Check sheet for the modelled part. Datum: model origin and axes. Units: mm. Face numbers are marked on the shaded views. A direction names the side the tool comes from. Give positions to 0.01 mm unless a question says otherwise; leave off trailing zeros. Loops run counter-clockwise (first coordinate to the right, second up) from the corner with the lowest first, then second, coordinate; pieces in that order, holes last. Notation, with made-up numbers: (54, 66) - (97, 66) arc R23 cw to (97, 74) - close; hole circle Ø7 at (-31, -24). An arc over 180 degrees is marked (long way). Answer in a Markdown table with one row per item. Add a question column.
(1) Set-up check for the marked faces 1 and 2: record each of +Z, -Z, +X, -X, +Y, -Y from which the full face is reachable in a straight line by a thin tool's end or side.
(2) Sectioned sample at A-A on y = 75. Enter the section's corners in (x, z).
(3) Go/stop test with flat-tipped pins: P1, Ø3, axis at x = 37.5, z = -37.5, coming from the +Y side; P2, Ø10, axis at x = 13.5, y = 96.5, coming from the +Z side; P3, Ø2.5, axis at x = 2.24, z = -37.13, coming from the +Y side. Record where each tip stops, or that it passes through.
(4) Sectioned sample at B-B on z = -2.5. Enter the section's corners in (x, y), then the cut area to 3 significant figures.
(5) Thickness scan on L1, parallel to Y at x = 15, z = -10; L2, parallel to Y at x = 15, z = -26.5; L3, parallel to X at y = 95, z = -20. Record the ranges inside material, lowest first.
(6) Sectioned sample at C-C on y = 91.5. Enter the section's corners in (x, z) (3 decimals).
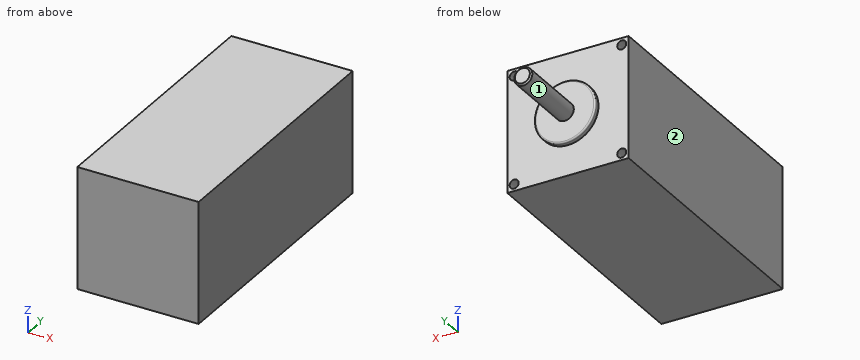
from build123d import *

# Parameters (mm, degrees)
SKETCH1_W      = 39.37
SKETCH1_H      = 85.852
EXTRUDE1_DEPTH = 39.37
SKETCH2_R      = 2.9337
EXTRUDE2_DEPTH = 25.4
CHAMFER1_SIZE  = 0.508
SKETCH4_R      = 9.906
EXTRUDE3_DEPTH = 1.778
FILLET3_R      = 0.508
SKETCH5_R      = 1.4605
EXTRUDE4_DEPTH = 12.7


with BuildPart() as part:
    # Sketch1 → Extrude1 (new body)
    with BuildSketch(Plane.XY):
        with Locations((19.685, 42.926)):
            Rectangle(SKETCH1_W, SKETCH1_H)
    extrude(amount=-EXTRUDE1_DEPTH)

    # Sketch2 → Extrude2 (add)
    with BuildSketch(Plane(origin=(0, 85.852, 0), x_dir=(1, 0, 0), z_dir=(0, 1, 0))):
        with Locations(Location((19.685, 19.685, 0), (0, 0, 270))):
            Circle(SKETCH2_R)
    extrude(amount=EXTRUDE2_DEPTH)

    # Chamfer1
    chamfer1_edges = [part.edges().sort_by_distance(p)[0] for p in [
        (19.685, 111.252, -22.6187),
    ]]
    chamfer(chamfer1_edges, length=CHAMFER1_SIZE)

    # Sketch4 → Extrude3 (add)
    with BuildSketch(Plane(origin=(0, 85.852, 0), x_dir=(1, 0, 0), z_dir=(0, 1, 0))):
        with Locations(Location((19.685, 19.685, 0), (0, 0, 270))):
            Circle(SKETCH4_R)
    extrude(amount=EXTRUDE3_DEPTH)

    # Fillet3
    fillet3_edges = [part.edges().sort_by_distance(p)[0] for p in [
        (19.685, 87.63, -29.591),
    ]]
    fillet(fillet3_edges, radius=FILLET3_R)

    # Sketch5 → Extrude4 (cut)
    with BuildSketch(Plane(origin=(0, 85.852, 0), x_dir=(1, 0, 0), z_dir=(0, 1, 0))):
        with Locations(Location((2.236362357, 37.133637643, 0), (0, 0, 270))):
            Circle(SKETCH5_R)
        with Locations(Location((37.133637643, 37.133637643, 0), (0, 0, 270))):
            Circle(SKETCH5_R)
        with Locations(Location((37.133637643, 2.236362357, 0), (0, 0, 270))):
            Circle(SKETCH5_R)
        with Locations(Location((2.236362357, 2.236362357, 0), (0, 0, 270))):
            Circle(SKETCH5_R)
    extrude(amount=-EXTRUDE4_DEPTH, mode=Mode.SUBTRACT)


solid = part.part
Reply:
| question | item | result |
|---|---|---|
| 1 | face 1 | +Y |
| 1 | face 2 | +Z, -Z, -X, +Y, -Y |
| 2 | outline | (0, -39.37) - (39.37, -39.37) - (39.37, 0) - (0, 0) - close; hole circle Ø2.92 at (2.24, -37.13); hole circle Ø2.92 at (2.24, -2.24); hole circle Ø2.92 at (37.13, -37.13); hole circle Ø2.92 at (37.13, -2.24) |
| 3 | P1 | y = 85.85 |
| 3 | P2 | z = -17 |
| 3 | P3 | y = 73.15 |
| 4 | outline | (0, 0) - (39.37, 0) - (39.37, 85.85) - (38.57, 85.85) - (38.57, 73.15) - (35.7, 73.15) - (35.7, 85.85) - (3.67, 85.85) - (3.67, 73.15) - (0.8, 73.15) - (0.8, 85.85) - (0, 85.85) - close |
| 4 | area | 3,310 mm^2 |
| 5 | L1 | 0 to 85.85 |
| 5 | L2 | 0 to 87.63 |
| 5 | L3 | 16.77 to 22.6 |
| 6 | outline | circle Ø5.867 at (19.685, -19.685) |
